from build123d import *

# Parameters (mm, degrees)
F0_R     = 7.5
F0_R_2   = 5.5
F1_DEPTH = 5
F2_DEPTH = 10
F3_SIZE  = 0.1


with BuildPart() as f1:
    # F0 (on Front) → F1 (new body)
    with BuildSketch(Plane.XZ):
        Circle(F0_R)
        Circle(F0_R_2, mode=Mode.SUBTRACT)
        Circle(F0_R_2)
    extrude(amount=-F1_DEPTH)

    # F0 (on Front) → F2 (join)
    with BuildSketch(Plane.XZ):
        Circle(F0_R_2)
    extrude(amount=F2_DEPTH)

    # F3
    f3_edges = [f1.edges().sort_by_distance(p)[0] for p in [
        (-5.5, -10, 0),
        (7.5, 2.5, 0),
        (-7.5, 0, 0),
        (-7.5, 5, 0),
    ]]
    chamfer(f3_edges, length=F3_SIZE)


solid = f1.part
Could you check a few things on this model? Use its own coordinates, in mm. A direction names the side the tool comes from. Give positions to 0.01 mm unless a question says otherwise; leave off trailing zeros. Order: outer loops, then holes, each group sorted by start corner. A loop starts at its lowest first (then second) coordinate and runs counter-clockwise, first axis right, second up.
1. Suppose I cut it at C-C (y = -5.5). List the corners of the cut face in (x, z) for me.
2. Suppose I cut it at A-A (z = 0). List the corners of the cut face in (x, y) for me, plus the area to 3 significant figures.
3. I need wall thicknesses on L1, parallel to Z at x = -1.25, y = 4; L2, parallel to Y at x = -5.5, z = -3; L3, parallel to Z at x = 6.25, y = 3.25. Which ranges of each line are inside material? Lowest first, please.
4. Will these pins go through, and if not, where does the flat tip stop? P1, Ø3, axis at x = 3.5, y = -5.5, coming from the +Z side; P2, Ø5, axis at y = 3, z = -3.5, coming from the +X side; P3, Ø2, axis at x = 4, y = -6.5, coming from the -Z side.
5. Suppose I cut it at B-B (x = 0). List the corners of the cut face in (y, z) for me, plus the area to 3 significant figures.
6. For faces 1 (the flat face through (0, -10, 0)), 2 (the flat face through (0, 0, 6)), which set-ups out of +Z, -Z, +X, -X, +Y, -Y let a thin tool reach every point of the face, with its end or its side?
7. Suppose I cut it at D-D (y = 3.5). List the corners of the cut face in (x, z) for me.
Solved:
1. outline: circle Ø11 at (0, 0)
2. outline: (-7.5, 0.1) - (-7.4, 0) - (-5.5, 0) - (-5.5, -9.9) - (-5.4, -10) - (5.4, -10) - (5.5, -9.9) - (5.5, 0) - (7.4, 0) - (7.5, 0.1) - (7.5, 4.9) - (7.4, 5) - (-7.4, 5) - (-7.5, 4.9) - close
2. area: 185 mm2
3. L1: z = -7.4 to 7.4
3. L2: y = 0 to 5
3. L3: z = -4.15 to 4.15
4. P1: stops at z = 5.12
4. P2: stops at x = 7.43
4. P3: stops at z = -4.61
5. outline: (-10, -5.4) - (-9.9, -5.5) - (0, -5.5) - (0, -7.4) - (0.1, -7.5) - (4.9, -7.5) - (5, -7.4) - (5, 7.4) - (4.9, 7.5) - (0.1, 7.5) - (0, 7.4) - (0, 5.5) - (-9.9, 5.5) - (-10, 5.4) - close
5. area: 185 mm2
6. face 1: +Z, -Z, +X, -X, -Y
6. face 2: -Y
7. outline: circle Ø15 at (0, 0)
